Input: part model. Units: mm. Frame: model coordinates. A direction names the side the tool comes from. Give positions to 0.01 mm unless a question says otherwise; leave off trailing zeros. Write each loop counter-clockwise with the first axis right and the second up, starting at its lowest first coordinate (ties: lowest second). Pieces come first, ordered by that corner, then holes. Notation, with made-up numbers: (69, 88) -> (126, 88) arc R19 cw to (126, 124) -> close; hole circle Ø2 at (16, 49). An arc over 180 degrees is marked (long way). Answer as a JSON object with one key per item and string values. Group by question number.
from build123d import *

# Parameters (mm, degrees)
F2_R      = 12.7
F5_R      = 2.54
F10_W     = 0.396875
F10_H     = 4.856163
F10_W_2   = 4.856162
F10_H_2   = 0.396875
F10_H_3   = 4.856162
F11_DEPTH = 12.7


with BuildPart() as f1:
    # F0 (on Front) → F1 (revolve)
    with BuildSketch(Plane.XZ):
        Polygon((-9.144, -33.673599), (0, -33.673599), (0, 42.526401), (-2.5654, 42.526401), (-9.144, 30.708205), (-9.144, 11.243628), (-4.7625, 0), align=None)
    revolve(axis=Axis((0, 0, 4.426401), (0, 0, 1)))

    # F2
    f2_edges = [f1.edges().sort_by_distance(p)[0] for p in [
        (9.144, 0, 30.708205),
    ]]
    fillet(f2_edges, radius=F2_R)

    # F3 (on Front) → F4 (revolve, cut)
    with BuildSketch(Plane.XZ):
        Polygon((0, -36.217926), (0, 0), (-3.161618, 0), (-7.874178, -36.217926), align=None)
    revolve(axis=Axis((0, 0, -18.108963), (0, 0, -1)), mode=Mode.SUBTRACT)

    # F5
    f5_edges = [f1.edges().sort_by_distance(p)[0] for p in [
        (3.161618, 0, 0),
    ]]
    fillet(f5_edges, radius=F5_R)

    # F6 (on Front) → F7 (revolve, cut)
    with BuildSketch(Plane.XZ):
        Polygon((0, -36.17549), (0, 0), (-3.188173, -12.631214), (-5.986212, -15.556437), (-8.669097, -36.17549), align=None)
    revolve(axis=Axis((0, 0, -18.087745), (0, 0, -1)), mode=Mode.SUBTRACT)

    # F8 (on Front) → F9 (revolve, cut)
    with BuildSketch(Plane.XZ):
        Polygon((0, 4.207624), (0, 46.769504), (-2.216791, 43.152663), (-2.216791, 38.256735), (-6.76275, 30.090099), (-6.76275, 11.691208), (-3.846492, 4.207624), align=None)
    revolve(axis=Axis((0, 0, 25.488564), (0, 0, -1)), mode=Mode.SUBTRACT)

    # F10 (on face) → F11 (cut)
    with BuildSketch(Plane.XY.offset(42.526401)):
        with Locations((1e-06, 2.626518)):
            Rectangle(F10_W, F10_H)
        Polygon((-0.198437, -0.198438), (-0.198437, 0.198437), (-5.0546, 0.198437), (-5.0546, -0.198437), align=None)
        with Locations((2.626519, -1e-06)):
            Rectangle(F10_W_2, F10_H_2)
        with Locations((1e-06, -2.626519)):
            Rectangle(F10_W, F10_H_3)
    extrude(amount=-F11_DEPTH, mode=Mode.SUBTRACT)


solid = f1.part
1. Line query: line 1 (Y direction, x = 0, z = 22); line 2 (Y direction, x = 2.25, z = -16); line 3 (Y direction, x = 4, z = -6). Output: solid intervals per line, ascending.
2. Section A-A (z = 8.5). Return the cut outline in (x, y).
3. Contact query for flat-ended pins moving along their axis: pin 1 Ø3 at (x, z) = (-6, -6.5) entering from +Y; pin 2 Ø0.9 at (y, z) = (4, 37.5) entering from +X; pin 3 Ø0.9 at (x, z) = (-4, 37) entering from -Y. Output: stop coordinate, or through.
4. Reachability of faces 4 (the face through (0.198, -4, 38)), 5 (the face through (-1.65, -1.73, 42.526)), 6 (the face through (0, 0, 0)), 7 (the face through (-3.35, 1.05, 35.93)) from +Z, -Z, +X, -X, +Y, -Y: full face, straight path, thin tool, end or side. Return the list, or none.
5. Section B-B (z = -6.5). Return the cut outline in (x, y).
6. Mould query, pull axis X, two halves, no side actions, for faces 1 (the face through (-8, 3, -33.674)), 2 (the face through (1.51, 6.82, -17.07)), 3 (the face through (4, 0.198, 38)). Classes: pulls with the +X half, pulls with the -X half, needs draft (parallel to the pull), parting line crosses it, or undercut.
Working result:
{
 "1": {"line 1": "y = -9.14 to -6.76, 6.76 to 9.14", "line 2": "y = -6.46 to -5.61, 5.61 to 6.46", "line 3": "y = -3.84 to 3.84"},
 "2": {"outline": "circle Ø16.15 at (0, 0); hole circle Ø11.04 at (0, 0)"},
 "3": {"pin 1": "stops at y = 3.37", "pin 2": "stops at x = 4.14", "pin 3": "stops at y = -4.51"},
 "4": {"face 4": "+Z", "face 5": "+Z, +X, -X, +Y, -Y", "face 6": "-Z", "face 7": "none"},
 "5": {"outline": "circle Ø11.22 at (0, 0); hole circle Ø8.01 at (0, 0)"},
 "6": {"face 1": "needs draft", "face 2": "parting line crosses it", "face 3": "undercut"}
}
